Autodesk Inventor part; units mm, degrees
ref_plane "YZ Plane" through (0, 0, 0) normal (1, 0, 0) x (0, 1, 0)
ref_plane "XZ Plane" through (0, 0, 0) normal (0, 1, 0) x (-1, 0, 0)
ref_plane "XY Plane" through (0, 0, 0) normal (0, 0, 1) x (1, 0, 0)
sketch "Sketch1" plane through (0, 0, 0) normal (0, 0, 1) x (1, 0, 0)
  line L0 (0, 8.9678) -> (0, -21.984)
  line L1 (-55.9342, 0) -> (8.6032, 0)
  circle A0 centre (-8.75, 0) radius 1.6
  circle A1 centre (8.75, 0) radius 1.6
  line L2 (-13, 27.4955) -> (13, 27.4955)
  line L3 (13, 27.4955) -> (13, -20.0499)
  line L4 (-13, -20.0499) -> (-13, 27.4955)
  circle A2 centre (0, 21.5844) radius 1
  circle A3 centre (0, 6.5844) radius 1
  circle A4 centre (0, -20.0499) radius 3.5
  line L5 (0, -20.0499) -> (8.75, 0)
  arc A5 (-13, -20.0499) -> (13, -20.0499) centre (0, -20.0499) ccw
  line L6 (-13, 2.4955) -> (-33, 2.4955)
  line L7 (-33, 2.4955) -> (-33, -2.5045)
  line L8 (-33, -2.5045) -> (-13, -2.5045)
  line L9 (13, 2.4955) -> (33, 2.4955)
  line L10 (33, 2.4955) -> (33, -2.5045)
  line L11 (33, -2.5045) -> (13, -2.5045)
  point P0 (0, 0)
  point P1 (-13, -2.5045)
  dimension "d1" = 17.5
  dimension "d2" = 3.2
  dimension "d3" = 15
  dimension "d4" = 2
  dimension "d7" = 26
  dimension "d8" = 7
  dimension "d9" = 21.876
  dimension "d14" = 5
  dimension "d15" = 20
  dimension "d22" = 25
extrude "Extrusion1" add sketch "Sketch1" along normal blind 3 contours L1 A1 L5 A4 L0 | L7 L6 L4 L1 | L1 L4 L8 L7 | L4 L2 L3 A5 | L3 L9 L10 L11
sketch "Sketch2" plane through (0, 0, 0) normal (0, 0, -1) x (-1, 0, 0)
  circle A0 centre (-8.75, 0) radius 1.6
  circle A1 centre (-8.75, 0) radius 1.6
  circle A2 centre (8.75, 0) radius 1.6
  circle A3 centre (8.75, 0) radius 1.6
  point P0 (0, 0)
extrude "Extrusion2" add sketch "Sketch2" along normal blind 10 and the other way blind 3
sketch "Sketch3" plane through (-33, 2.4955, 0) normal (0, 1, 0) x (1, 0, 0)
  circle A0 centre (7.5, -0.5) radius 2.5
  line L0 (20, 0) -> (0, 0)
  line L1 (0, 0) -> (0, -3)
  line L2 (0.0505, -3) -> (0, -3)
  line L3 (0, -3) -> (0, 0)
  line L4 (0, 0) -> (9.9495, 0)
  line L5 (20, -3) -> (0, -3)
  point P0 (33, 0)
  point P1 (5.1646, -1.3921)
  dimension "d16" = 5
  dimension "d26" = 7.5
extrude "Extrusion3" add sketch "Sketch3" along normal blind 7 contours A0 L0 | L0 A0
fillet "Fillet1" radius 2 2 edges at (10.35, 0, 0) (-7.15, 0, 0)
fillet "Fillet2" radius 1.9 1 edges at (-25.5, 2.4955, 0)
mirror "Mirror1" about plane through (0, 0, 0) normal (1, 0, 0) of "Extrusion3"
mirror "Mirror3" about plane through (0, 0, 0) normal (1, 0, 0) of "Fillet2"
sketch "Sketch5" plane through (25.5, 9.4955, 0.5) normal (0, 1, 0) x (1, 0, 0)
  circle A0 centre (0, 0) radius 5
  line L0 (-12.5, -2.5) -> (7.5, -2.5)
  line L1 (4.3301, -2.5) -> (9.1307, -2.5)
  line L2 (9.1307, -2.5) -> (9.1307, 0.5)
  line L3 (9.1307, 0.5) -> (4.9749, 0.5)
  line L4 (-12.5, 0.5) -> (7.5, 0.5)
  point P0 (-25.5, 0.5)
  dimension "d27" = 10
extrude "Extrusion5" cut sketch "Sketch5" against normal up to surface (12 mm away) contours A0 L3 L2 L1 L0
mirror "Mirror4" about plane through (0, 0, 0) normal (1, 0, 0) of "Extrusion5"
properties part number "pintutucu"
Geometry check sheet. Reference: the model listing, model coordinates, mm. A direction names the side the tool comes from. Round coordinates to 2 decimals unless told otherwise and drop trailing zeros. Loops run counter-clockwise (first coordinate to the right, second up) from the corner with the lowest first, then second, coordinate; pieces in that order, holes last.
Item 1: Cross-section at B-B on z = -7.5. Record the boundary of the cut face in (x, y).
Item 2: Cross-section at C-C on x = 8.75. Record the boundary of the cut face in (y, z), then the cut area to 3 significant figures.
Item 3: Cross-section at D-D on y = 13. Record the boundary of the cut face in (x, z), then the cut area to 3 significant figures.
Item 4: Access from +Z, -Z, +X, -X, +Y, -Y to the whole of each face (thin tool, end or side, straight path). Record for faces 4 (the cylindrical face through (10.35, -0.07, -5.94)), 5 (the flat face through (-13, -11, 1)), 6 (the flat face through (-13, 15, 1)), 7 (the flat face through (25, 9.496, 0)).
Item 5: Thickness scan on line 1 (Y direction, x = 0, z = 2.3); line 2 (Z direction, x = 7, y = 6.5); line 3 (X direction, y = -11, z = 1.5). Record the ranges inside material, lowest first.
Item 6: Gauge pin test, flat ends, axial feed: pin 1 (2.5 mm diameter, centred on x = 27, z = 1, fed in from +Y); pin 2 (6 mm diameter, centred on x = 21.5, y = 8, fed in from +Z); pin 3 (0.9 mm diameter, centred on x = 21, z = 2, fed in from -Y); pin 4 (6 mm diameter, centred on x = -14.5, z = 1, fed in from +Y). Record the tip position at first contact, or that the pin passes through.
Item 7: Mould release check, pull along X, two halves, no side actions. Record for faces 1 (the cylindrical face through (-0.22, 7.56, 1.48)), 2 (the flat face through (-26, 9.496, 0)), 3 (the cylindrical face through (0.286, -33.047, 1.479)): pulls with the +X half, pulls with the -X half, needs draft (parallel to the pull), parting line crosses it, or undercut.
Item 8: Cross-section at A-A on x = 0. Record the boundary of the cut face in (y, z).
Answer sheet:
1. outline: circle Ø3.2 at (-8.75, 0); circle Ø3.2 at (8.75, 0)
2. outline: (-29.66, 0) - (-3.6, 0) arc R2 cw to (-1.6, -2) - (-1.6, -10) - (1.6, -10) - (1.6, -2) arc R2 cw to (3.6, 0) - (27.5, 0) - (27.5, 3) - (-29.66, 3) - close
2. area: 205 mm2
3. outline: (-13, 0) - (13, 0) - (13, 3) - (-13, 3) - close
3. area: 78.0 mm2
4. face 4: -Z
4. face 5: +Z, -Z, -X, -Y
4. face 6: +Z, -Z, +Y
4. face 7: +Z, -Z, +X, +Y
5. line 1: y = -33.05 to -23.55, -16.55 to 5.58, 7.58 to 20.58, 22.58 to 27.5
5. line 2: z = 0 to 3
5. line 3: x = -13 to 13
6. pin 1: stops at y = 9.5
6. pin 2: stops at z = 2.79
6. pin 3: stops at y = -2.5
6. pin 4: stops at y = 27.5
7. face 1: undercut
7. face 2: needs draft
7. face 3: parting line crosses it
8. outline: (-33.05, 0) - (-23.55, 0) - (-23.55, 3) - (-33.05, 3) - close; (-16.55, 0) - (5.58, 0) - (5.58, 3) - (-16.55, 3) - close; (7.58, 0) - (20.58, 0) - (20.58, 3) - (7.58, 3) - close; (22.58, 0) - (27.5, 0) - (27.5, 3) - (22.58, 3) - close
